Model file for the job. Use its own axes, mm. A direction names the side the tool comes from. Coordinates: 2 decimals unless noted, no trailing zeros. Write each loop counter-clockwise with the first axis right and the second up, starting at its lowest first coordinate (ties: lowest second). Pieces come first, ordered by that corner, then holes. Notation, with made-up numbers: M -13,35 L 35,35 A27 ccw 35,63 Z; hole C 58.5,15 d4. An arc over 180 degrees is marked long. One line per question, with ' | ' between items. Start each with the question number.
(1) Cut at B-B (x = 12.25). Write the cut outline in (y, z) (3 decimals), plus the area to 3 significant figures.
(2) Cut at D-D (z = -2.25). Write the cut outline in (x, y), plus the area to 3 significant figures.
(3) Tool access for faces 5 (the face through (22.18, 14.83, -11.99)), 6 (the face through (9, 15, -18.415)), 7 (the face through (9, 16.891, -22)), 8 (the face through (9, 13.716, -5)): list every direction of +Z, -Z, +X, -X, +Y, -Y with a clear straight run to the whole face (end or side of a thin tool).
(4) Flat gauge pins, fed straight in: pin 1 Ø6 at (x, z) = (18.5, -20.5) entering from +Y; pin 2 Ø9.5 at (x, z) = (12, -17) entering from +Y; pin 3 Ø3 at (y, z) = (18.5, -8) entering from -X. Where does each tip first touch, or does it go through?
(5) Wall check: probe 1 along Y at (x, z) = (23.25, -12.7); probe 2 along Y at (x, z) = (18.75, -4.5); probe 3 along Z at (x, y) = (4, 13.5) (3 decimals). Give the ranges that are in metal, low to high.
(6) Two-plate mould, pull along Y, no slides. Class faces 1 (the face through (13, 0, -13)), 2 (the face through (9, 15, -6.985)), 3 (the face through (9, 12, -3.175)), 4 (the face through (22, 20.701, -13)): +Y half, -Y half, draft (parallel to the pull), parting line (faces both ways), or undercut.
(7) Cut at A-A (z = -12.7). Write the cut outline in (x, y), plus the area to 3 significant figures.
(8) Cut at C-C (y = 14.5). Write the cut outline in (x, z) (3 decimals), plus the area to 3 significant figures.
Autodesk Inventor part; units mm, degrees
ref_plane "YZ Plane" through (0, 0, 0) normal (1, 0, 0) x (0, 1, 0)
ref_plane "XZ Plane" through (0, 0, 0) normal (0, 1, 0) x (-1, 0, 0)
ref_plane "XY Plane" through (0, 0, 0) normal (0, 0, 1) x (1, 0, 0)
sketch "Sketch1" plane through (0, 0, 0) normal (1, 0, 0) x (0, 1, 0)
  line L0 (0, 0) -> (16.891, 0)
  line L1 (16.891, 0) -> (16.891, -25.4)
  line L2 (16.891, -25.4) -> (0, -25.4)
  line L3 (0, -25.4) -> (0, 0)
  line L4 (16.891, -6.985) -> (13.716, -6.985)
  line L5 (13.716, -6.985) -> (13.716, -3.175)
  line L6 (13.716, -3.175) -> (10.541, -3.175)
  line L7 (10.541, -3.175) -> (10.541, -22.225)
  line L8 (10.541, -22.225) -> (13.716, -22.225)
  line L9 (13.716, -22.225) -> (13.716, -18.415)
  line L10 (13.716, -18.415) -> (16.891, -18.415)
  dimension "d0" = 25.4
  dimension "d1" = 11.43
  dimension "d2" = 19.05
  dimension "d3" = 3.81
  dimension "d4" = 6.985
  dimension "d5" = 3.175
  dimension "d6" = 6.35
  dimension "d7" = 16.891
extrude "Extrusion1" add sketch "Sketch1" along normal blind 19.05 contours L0 L1 L4 L5 L6 L7 L8 L9 L10 L2 L3
sketch "Sketch2" plane through (19.05, 0, 0) normal (1, 0, 0) x (0, 0, -1)
  line L0 (0, 0) -> (25.4, 0)
  line L1 (25.4, 0) -> (25.4, 20.701)
  line L2 (25.4, 20.701) -> (0, 20.701)
  line L3 (0, 20.701) -> (0, 0)
  line L4 (25.4, 16.891) -> (18.415, 16.891)
  dimension "d10" = 3.81
  dimension "d11" = 25.4
extrude "Extrusion2" add sketch "Sketch2" along normal blind 6.35
sketch "Sketch4" plane through (19.05, 0, 0) normal (-1, 0, 0) x (0, 0, 1)
  circle A0 centre (-12.7, 13.716) radius 1.3208
  line L0 (0, 16.891) -> (0, 0)
  line L1 (-22.225, 10.541) -> (-3.175, 10.541)
  line L2 (-3.175, 13.716) -> (-6.985, 13.716)
  dimension "d21" = 2.6416
  dimension "d22" = 12.7
  dimension "d23" = 3.175
  dimension "d24" = 0
extrude "Extrusion3" cut sketch "Sketch4" against normal through all
equation "\"d3\" = -0.5 * d1 + 0.5 * d2"
equation "\"d4\" = -0.5 * d1 + 0.5 * d0"
properties part number "tenshoner base"
Filled in:
1) outline: M 0,-25.4 L 16.891,-25.4 L 16.891,-18.415 L 13.716,-18.415 L 13.716,-22.225 L 10.541,-22.225 L 10.541,-3.175 L 13.716,-3.175 L 13.716,-6.985 L 16.891,-6.985 L 16.891,0 L 0,0 Z | area: 332 mm²
2) outline: M 0,0 L 25.4,0 L 25.4,20.7 L 19.05,20.7 L 19.05,16.89 L 0,16.89 Z | area: 453 mm²
3) face 5: +X, -X | face 6: -X, +Y | face 7: +Z, -Z, -X, +Y | face 8: -X
4) pin 1: y = 20.7 | pin 2: y = 16.89 | pin 3: x = 19.05
5) probe 1: 0 to 12.4, 15.04 to 20.7 | probe 2: 0 to 10.54, 13.72 to 16.89 | probe 3: -25.4 to -22.225, -3.175 to 0
6) face 1: -Y half | face 2: draft | face 3: undercut | face 4: +Y half
7) outline: M 0,0 L 25.4,0 L 25.4,12.4 L 19.05,12.4 L 19.05,10.54 L 0,10.54 Z; M 19.05,15.04 L 25.4,15.04 L 25.4,20.7 L 19.05,20.7 Z | area: 315 mm²
8) outline: M 0,-25.4 L 25.4,-25.4 L 25.4,-13.763 L 19.05,-13.763 L 19.05,-18.415 L 0,-18.415 Z; M 0,-6.985 L 19.05,-6.985 L 19.05,-11.637 L 25.4,-11.637 L 25.4,0 L 0,0 Z | area: 414 mm²
